Can you work these out from the model? Positions are in its coordinate system, mm. A direction names the side the tool comes from. Give positions to 0.01 mm unless a question says otherwise; leave off trailing zeros. Loops run counter-clockwise (first coordinate to the right, second up) from the corner with the lowest first, then second, coordinate; pieces in that order, holes last. Notation, with made-up numbers: M 62,80.5 L 83,80.5 A13 ccw 83,92.5 Z; hole C -37.5,22 d4. An arc over 180 degrees is marked long. Use CSV: the item, a comma, the result in double quotes.
Autodesk Inventor part; units mm, degrees
ref_plane "YZ Plane" through (0, 0, 0) normal (1, 0, 0) x (0, 1, 0)
ref_plane "XZ Plane" through (0, 0, 0) normal (0, 1, 0) x (-1, 0, 0)
ref_plane "XY Plane" through (0, 0, 0) normal (0, 0, 1) x (1, 0, 0)
sketch "Boceto1" plane through (0, 0, 0) normal (0, 1, 0) x (-1, 0, 0)
  circle A0 centre (0, 0) radius 15
  circle A1 centre (0, 0) radius 75
  arc A2 (-10.6675, 21.8887) -> (10.6675, 21.8887) centre (0, 35.706) ccw
  arc A3 (21.8887, 10.6675) -> (10.6675, 21.8887) centre (15.5563, 15.5563) ccw
  arc A4 (21.8887, 10.6675) -> (21.8887, -10.6675) centre (35.706, 0) ccw
  arc A5 (10.6675, -21.8887) -> (21.8887, -10.6675) centre (15.5563, -15.5563) ccw
  arc A6 (10.6675, -21.8887) -> (-10.6675, -21.8887) centre (0, -35.706) ccw
  arc A7 (-21.8887, -10.6675) -> (-10.6675, -21.8887) centre (-15.5563, -15.5563) ccw
  arc A8 (-21.8887, -10.6675) -> (-21.8887, 10.6675) centre (-35.706, 0) ccw
  arc A9 (-10.6675, 21.8887) -> (-21.8887, 10.6675) centre (-15.5563, 15.5563) ccw
  circle A10 centre (0, -22.5) radius 1.5
  circle A11 centre (22.5, 0) radius 1.5
  circle A12 centre (0, 22.5) radius 1.5
  circle A13 centre (-22.5, 0) radius 1.5
  circle A14 centre (0, 0) radius 15.25
  dimension "d0" = 30
  dimension "d1" = 150
extrude "Extrusión1" add sketch "Boceto1" along normal blind 5 contours A1
properties part number "Plato T5"
Q1. I want a section at C-C, the plane z = 47. Please give me the cut outline in (x, y).
Model answer:
outline,"M -58.45,0 L 58.45,0 L 58.45,5 L -58.45,5 Z"
Q2. For faces 4 (the cylindrical face through (-18.25, 2.46, -0.16)), 5 (the flat face through (1, 5, -32)), which set-ups out of +Z, -Z, +X, -X, +Y, -Y let a thin tool reach every point of the face, with its end or its side?
Model answer:
face 4,"+Y, -Y"
face 5,"+Z, -Z, +X, -X, +Y"
Q3. I want a section at A-A, the plane y = 2.85. Please give me the cut outline in (x, z), then the cut area to 3 significant figures.
Model answer:
outline,"C 0,0 d150; hole C -22.5,0 d3; hole M -21.89,-10.67 A8 ccw -10.67,-21.89 A17.46 cw 10.67,-21.89 A8 ccw 21.89,-10.67 A17.46 cw 21.89,10.67 A8 ccw 10.67,21.89 A17.46 cw -10.67,21.89 A8 ccw -21.89,10.67 A17.46 cw Z; hole C 0,-22.5 d3; hole C 0,22.5 d3; hole C 22.5,0 d3"
area,"15,900 mm2"
Q4. If we mould it in two halves opening along Z, with no side actions, what happens to faces 1 (the cylindrical face through (-0.16, 2.46, 18.25)), 2 (the flat face through (1, 0, -32)), 3 (the cylindrical face through (9.764, 2.465, -74.362))? For each: released by +Z, released by -Z, zero draft, split by the parting line, or undercut.
Model answer:
face 1,"undercut"
face 2,"zero draft"
face 3,"split by the parting line"
Q5. I'm going to push flat-ended pins straight in: P1, Ø2, axis at y = 3.5, z = 12.5, coming from the -X side; P2, Ø2, axis at y = 4, z = 23, coming from the -X side; P3, Ø2, axis at y = 1, z = -33, coming from the -X side. Where does each tip first touch, or does it pass through?
Model answer:
P1,"x = -74.11"
P2,"x = -71.7"
P3,"x = -67.83"
Q6. Please list where these lines run through material, in increasing order: L1, parallel to Z at x = 22.5, y = 3.65; L2, parallel to X at y = 0.95, z = -12; L3, parallel to Z at x = -8, y = 2. Write a range as from..to.
Model answer:
L1,"-71.55..-19.53, -11.58..-1.5, 1.5..11.58, 19.53..71.55"
L2,"-74.03..-22.72, 22.72..74.03"
L3,"-74.57..-20.19, 20.19..74.57"
Q7. I want a section at B-B, the plane z = 62.5. Please give me the cut outline in (x, y).
Model answer:
outline,"M -41.46,0 L 41.46,0 L 41.46,5 L -41.46,5 Z"
